Verification items for the finished model (mm, model axes). Face numbers are marked on the shaded views. A direction names the side the tool comes from. Round coordinates to 2 decimals unless told otherwise and drop trailing zeros. Order: outer loops, then holes, each group sorted by start corner. A loop starts at its lowest first (then second) coordinate and runs counter-clockwise, first axis right, second up. Notation, with made-up numbers: (13.25, 20.25) -> (20.25, 20.25) arc R37 ccw to (20.25, 57.25) -> close; hole circle Ø10 at (13.25, 10). An arc over 180 degrees is marked (long way). Return JSON: item names as keys, results as strings. Group by question number.
1) Section check A-A on z = -5.5. Enter the section's corners in (x, y) (3 decimals), plus the area to 3 significant figures.
2) Depth check by flat-ended pin: pin 1 (4.5 mm diameter, centred on x = 193.68, z = -16.67, fed in from +Y); pin 2 (6 mm diameter, centred on x = 32, y = 6, fed in from -Z); pin 3 (1 mm diameter, centred on x = 124, y = 32.5, fed in from -Z). Enter the tip coordinate at first touch or a pass-through.
3) Scan lines: L1, parallel to Y at x = 146, z = -26.5 (3 decimals); L2, parallel to Z at x = 112.5, y = 13.5 (3 decimals); L3, parallel to Y at x = 85, z = -2.5. Record each from-to range of solid material in increasing order.
4) Section check B-B on x = 143. Enter the section's corners in (y, z) (3 decimals).
5) Section check C-C on y = 19. Enter the section's corners in (x, z) (3 decimals), plus the area to 3 significant figures.
6) Draft check along Y on the marked faces 1, 2, 3 and 4. Enter one of: pulls with the +Y half, pulls with the -Y half, needs draft (parallel to the pull), parting line crosses it, or undercut.
7) Tool access check on the marked faces 5 and 6. Record the directions out of +Z, -Z, +X, -X, +Y, -Y that give a thin tool (end or side, any length) a straight path to the whole face; none if there is none.
```python
from build123d import *

# Parameters (mm, degrees)
BASE_FLANGE1_DEPTH = 209.55
SKETCH6_R          = 3.3782
SKETCH6_R_2        = 2.4257
CUT_EXTRUDE1_DEPTH = 216.488725923
FILLET1_R          = 3.175


# Sheet-metal steps are written as plain solids
with BuildPart() as part:
    # Sketch1 → Base-Flange1 (new body)
    with BuildSketch(Plane(origin=(0, 0, 0), x_dir=(0, 0, -1), z_dir=(1, 0, 0))):
        with BuildLine():
            Line((30.226, 33.782), (3.175, 33.782))
            ThreePointArc((3.175, 33.782), (0.92993597, 32.85206403), (0, 30.607))
            Line((0, 30.607), (0, 3.175))
            ThreePointArc((0, 3.175), (0.92993597, 0.92993597), (3.175, 0))
            Line((3.175, 0), (30.226, 0))
            Line((30.226, 0), (30.226, -3.175))
            Line((30.226, -3.175), (3.175, -3.175))
            ThreePointArc((3.175, -3.175), (-1.315128061, -1.315128061), (-3.175, 3.175))
            Line((-3.175, 3.175), (-3.175, 30.607))
            ThreePointArc((-3.175, 30.607), (-1.315128061, 35.097128061), (3.175, 36.957))
            Line((3.175, 36.957), (30.226, 36.957))
            Line((30.226, 36.957), (30.226, 33.782))
        make_face()
    extrude(amount=BASE_FLANGE1_DEPTH)

    # Sketch6 → Cut-Extrude1 (cut, through all)
    with BuildSketch(Plane(origin=(0, 36.957, 0), x_dir=(1, 0, 0), z_dir=(0, 1, 0))):
        with Locations(Location((28.575, 16.66875, 0), (0, 0, 270))):
            Circle(SKETCH6_R)
        with Locations(Location((92.075, 16.66875, 0), (0, 0, 270))):
            Circle(SKETCH6_R_2)
        with Locations(Location((155.575, 16.66875, 0), (0, 0, 270))):
            Circle(SKETCH6_R_2)
        with Locations(Location((193.675, 16.66875, 0), (0, 0, 270))):
            Circle(SKETCH6_R_2)
    extrude(amount=-CUT_EXTRUDE1_DEPTH, mode=Mode.SUBTRACT)

    # Fillet1
    fillet1_edges = [part.edges().sort_by_distance(p)[0] for p in [
        (0, -1.5875, -30.226),
        (0, 35.3695, -30.226),
        (209.55, -1.5875, -30.226),
        (209.55, 35.3695, -30.226),
    ]]
    fillet(fillet1_edges, radius=FILLET1_R)


solid = part.part
```
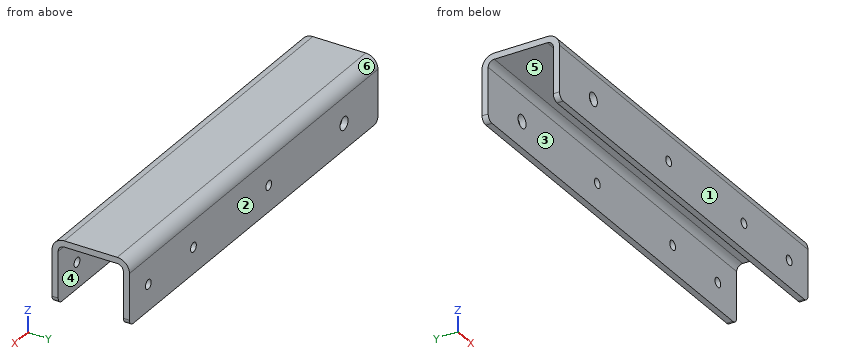
Check result:
{
 "1": {"outline": "(0, -3.175) -> (209.55, -3.175) -> (209.55, 0) -> (0, 0) -> close; (0, 33.782) -> (209.55, 33.782) -> (209.55, 36.957) -> (0, 36.957) -> close", "area": "1,330 mm^2"},
 "2": {"pin 1": "through", "pin 2": "z = 0", "pin 3": "z = -1.09"},
 "3": {"L1": "-3.175 to 0, 33.782 to 36.957", "L2": "0 to 3.175", "L3": "-3.14 to 0.07, 33.71 to 36.92"},
 "4": {"outline": "(-3.175, -30.226) -> (0, -30.226) -> (0, -3.175) arc R3.175 cw to (3.175, 0) -> (30.607, 0) arc R3.175 cw to (33.782, -3.175) -> (33.782, -30.226) -> (36.957, -30.226) -> (36.957, -3.175) arc R6.35 ccw to (30.607, 3.175) -> (3.175, 3.175) arc R6.35 ccw to (-3.175, -3.175) -> close"},
 "5": {"outline": "(0, 0) -> (209.55, 0) -> (209.55, 3.175) -> (0, 3.175) -> close", "area": "665 mm^2"},
 "6": {"face 1": "pulls with the -Y half", "face 2": "pulls with the +Y half", "face 3": "undercut", "face 4": "undercut"},
 "7": {"face 5": "-Z, +X, -X", "face 6": "+Z, +X, -X, +Y"}
}
